```python
from build123d import *

# Parameters (mm, degrees)
SKETCH_3_R          = 1.65
EXTRUDE_2_DEPTH     = 3
SKETCH_4_W          = 4
SKETCH_4_H          = 35.070805957
SKETCH_4_R          = 1.25
EXTRUDE_3_DEPTH     = 4
CUT_EXTRUDE_START   = -10
SKETCH_5_R          = 1
SKETCH_5_R_2        = 1.25
CUT_EXTRUDE_1_DEPTH = 10
FILLET_1_R          = 3
FILLET_2_R          = 3
FILLET_3_R          = 3
FILLET_4_R          = 3


with BuildPart() as part:
    # 草图3 → 凸台-拉伸2 (new body)
    with BuildSketch(Plane.XY):
        Polygon((-35.565841924, 57.58934902), (-72.610989278, 57.58934902), (-73.610989278, 57.58934902), (-73.610989278, 22.518543063), (-72.610989278, 22.518543063), (-35.565841924, 22.518543063), (-34.565841924, 22.518543063), (-34.565841924, 57.58934902), align=None)
        with Locations((-56.974581146, 28.517016942)):
            Circle(SKETCH_3_R, mode=Mode.SUBTRACT)
        with Locations((-65.61538335, 36.843873328)):
            Circle(SKETCH_3_R, mode=Mode.SUBTRACT)
        with Locations((-45.44291088, 31.836742967)):
            Circle(SKETCH_3_R, mode=Mode.SUBTRACT)
        with Locations((-62.724515288, 48.490455739)):
            Circle(SKETCH_3_R, mode=Mode.SUBTRACT)
        with Locations((-42.552042818, 43.483325377)):
            Circle(SKETCH_3_R, mode=Mode.SUBTRACT)
        with Locations((-51.192845022, 51.810181763)):
            Circle(SKETCH_3_R, mode=Mode.SUBTRACT)
    extrude(amount=EXTRUDE_2_DEPTH)

    # 草图4 → 凸台-拉伸3 (add)
    # profile 1 of 2: a face of its own
    with BuildSketch(Plane.XY.offset(3)):
        with Locations((-71.610989278, 40.053946041)):
            Rectangle(SKETCH_4_W, SKETCH_4_H)
        with Locations((-71.610989278, 47.08934902)):
            Circle(SKETCH_4_R, mode=Mode.SUBTRACT)
        with Locations((-71.610989278, 33.018543063)):
            Circle(SKETCH_4_R, mode=Mode.SUBTRACT)
        with Locations((-71.610989278, 40.053946042)):
            Circle(SKETCH_4_R, mode=Mode.SUBTRACT)
    # profile 2 of 2: a face of its own
    with BuildSketch(Plane.XY.offset(3)):
        with Locations((-36.565841924, 40.053946041)):
            Rectangle(SKETCH_4_W, SKETCH_4_H)
        with Locations((-36.565841924, 47.08934902)):
            Circle(SKETCH_4_R, mode=Mode.SUBTRACT)
        with Locations((-36.565841924, 40.053946042)):
            Circle(SKETCH_4_R, mode=Mode.SUBTRACT)
        with Locations((-36.565841924, 33.018543063)):
            Circle(SKETCH_4_R, mode=Mode.SUBTRACT)
    extrude(amount=EXTRUDE_3_DEPTH)

    # 草图5 → 切除-拉伸1 (cut)
    with BuildSketch(Plane.XY.offset(3).offset(CUT_EXTRUDE_START)):
        with Locations((-54.083713084, 40.163599353)):
            Circle(SKETCH_5_R)
        with Locations((-71.610989278, 47.08934902)):
            Circle(SKETCH_5_R_2)
        with Locations((-71.610989278, 40.053946042)):
            Circle(SKETCH_5_R_2)
        with Locations((-71.610989278, 33.018543063)):
            Circle(SKETCH_5_R_2)
        with Locations((-36.565841924, 47.08934902)):
            Circle(SKETCH_5_R_2)
        with Locations((-36.565841924, 40.053946042)):
            Circle(SKETCH_5_R_2)
        with Locations((-36.565841924, 33.018543063)):
            Circle(SKETCH_5_R_2)
    extrude(amount=CUT_EXTRUDE_1_DEPTH, mode=Mode.SUBTRACT)

    # 圆角1
    fillet_1_edges = [part.edges().sort_by_distance(p)[0] for p in [
        (-73.610989278, 22.518543063, 3.5),
    ]]
    fillet(fillet_1_edges, radius=FILLET_1_R)

    # 圆角2
    fillet_2_edges = [part.edges().sort_by_distance(p)[0] for p in [
        (-73.610989278, 57.58934902, 3.5),
    ]]
    fillet(fillet_2_edges, radius=FILLET_2_R)

    # 圆角3
    fillet_3_edges = [part.edges().sort_by_distance(p)[0] for p in [
        (-34.565841924, 57.58934902, 3.5),
    ]]
    fillet(fillet_3_edges, radius=FILLET_3_R)

    # 圆角4
    fillet_4_edges = [part.edges().sort_by_distance(p)[0] for p in [
        (-34.565841924, 22.518543063, 3.5),
    ]]
    fillet(fillet_4_edges, radius=FILLET_4_R)


solid = part.part
```
Geometry: final body of the model. Coordinates: model frame, mm. A direction names the side the tool comes from. Coordinates: 2 decimals unless noted, no trailing zeros. Order: outer loops, then holes, each group sorted by start corner. A loop starts at its lowest first (then second) coordinate and runs counter-clockwise, first axis right, second up.
Item 1: Contact query for flat-ended pins moving along their axis: P1, Ø1, axis at x = -61.5, y = 34, coming from the -Z side; P2, Ø2, axis at x = -36.57, y = 40.05, coming from the -Z side; P3, Ø4.5, axis at x = -62.72, y = 48.49, coming from the +Z side. Output: stop coordinate, or through.
Answer:
P1: stops at z = 0
P2: passes through
P3: stops at z = 3
Item 2: Section query D-D (z = 1.75). State how many separate pieces and enclosed holes the cut face has, then the cut area to 3 significant figures.
Answer:
separate pieces: 1
enclosed holes: 13
area: 1,280 mm2
Item 3: Section query B-B (y = 54). Output: boundary loops of the cut face in (x, z), then the cut area to 3 significant figures.
Answer:
outline: (-73.61, 0) - (-34.57, 0) - (-34.57, 7) - (-38.57, 7) - (-38.57, 3) - (-69.61, 3) - (-69.61, 7) - (-73.61, 7) - close
area: 149 mm2
Item 4: Section query A-A (z = 3.75). Output: boundary loops of the cut face in (x, y), then the cut area to 3 significant figures.
Answer:
outline: (-73.61, 25.52) arc R3 ccw to (-70.61, 22.52) - (-69.61, 22.52) - (-69.61, 57.59) - (-70.61, 57.59) arc R3 ccw to (-73.61, 54.59) - close; (-38.57, 22.52) - (-37.57, 22.52) arc R3 ccw to (-34.57, 25.52) - (-34.57, 54.59) arc R3 ccw to (-37.57, 57.59) - (-38.57, 57.59) - close; hole circle Ø2.5 at (-71.61, 33.02); hole circle Ø2.5 at (-71.61, 40.05); hole circle Ø2.5 at (-71.61, 47.09); hole circle Ø2.5 at (-36.57, 33.02); hole circle Ø2.5 at (-36.57, 40.05); hole circle Ø2.5 at (-36.57, 47.09)
area: 243 mm2
Item 5: Draft query along Y for faces 1 (the face through (-54, 22.519, 1)), 2 (the face through (-49.67, 51.18, 1.48)), 3 (the face through (-72.756, 56.687, 3.549)), 4 (the face through (-54, 36, 0)). Return one class per face: released by +Y, released by -Y, zero draft, split by the parting line, or undercut.
Answer:
face 1: released by -Y
face 2: undercut
face 3: released by +Y
face 4: zero draft
Item 6: Section query C-C (x = -41.5). Output: boundary loops of the cut face in (y, z).
Answer:
outline: (22.52, 0) - (42.21, 0) - (42.21, 3) - (22.52, 3) - close; (44.75, 0) - (57.59, 0) - (57.59, 3) - (44.75, 3) - close
Item 7: Material intervals for line 1 along X through (y, z) = (45, 4.5); line 2 along X through (y, z) = (39, 1.5); line 3 along Y through (x, z) = (-71.5, 6.5), sorted ascending.
Answer:
line 1: x = -73.61 to -69.61, -38.57 to -34.57
line 2: x = -73.61 to -72.28, -70.94 to -37.24, -35.89 to -34.57
line 3: y = 22.65 to 31.77, 34.26 to 38.81, 41.3 to 45.84, 48.33 to 57.45
Item 8: Access query for faces 5 (the face through (-35.41, 32.54, 3.45)), 6 (the face through (-69.611, 40, 5)). Directions: +Z, -Z, +X, -X, +Y, -Y. A direction counts if a zero-diameter tool reaches every point of the face in a straight line with its end or side. Return the directions, or none.
Answer:
face 5: +Z, -Z
face 6: +Z, +Y, -Y
